Verification items for the finished model (mm, model axes). Face numbers are marked on the shaded views. A direction names the side the tool comes from. Coordinates: 2 decimals unless noted, no trailing zeros. Order: outer loops, then holes, each group sorted by start corner. A loop starts at its lowest first (then second) coordinate and runs counter-clockwise, first axis right, second up. Notation, with made-up numbers: (-9, -16) -> (15, -16) arc R12 cw to (15, -3) -> close; hole circle Ø5 at (80.5, 84.25). An arc over 180 degrees is marked (long way). Use CSV: the item, a comma, the result in double quotes. Start each with the question number.
1) Sectioned sample at D-D on z = -24. Record the boundary of the cut face in (x, y) (3 decimals).
2) Go/stop test with flat-tipped pins: pin 1 (4 mm diameter, centred on x = -39.5, y = 5.5, fed in from +Z); pin 2 (6.5 mm diameter, centred on x = -28, y = 9, fed in from -Z); pin 3 (19 mm diameter, centred on x = -19, z = -33.5, fed in from -Y); pin 4 (2 mm diameter, centred on x = -34, y = 9, fed in from -Z). Record where each tip stops, or that it passes through.
3) Release check for a two-part mould opening along X. For the marked faces 6, 7 and 8 record: released by +X, released by -X, zero draft, split by the parting line, or undercut.
4) Sectioned sample at A-A on z = 2.5. Record the boundary of the cut face in (x, y) (3 decimals), then the cut area to 3 significant figures.
5) Sectioned sample at C-C on y = 14. Record the boundary of the cut face in (x, z) (3 decimals), then the cut area to 3 significant figures.
6) Scan lines: line 1 along X through (y, z) = (8, -3) (3 decimals); line 2 along X through (y, z) = (8, 3.5) (3 decimals); line 3 along Y through (x, z) = (-34.5, -59.5) (3 decimals). Record each from-to range of solid material in increasing order.
7) Sectioned sample at B-B on x = -18. Record the boundary of the cut face in (y, z) (1 decimal).
8) Tool access check on the marked faces 1, 2, 3, 4 and 5. Record the directions out of +Z, -Z, +X, -X, +Y, -Y that give a thin tool (end or side, any length) a straight path to the whole face; none if there is none.
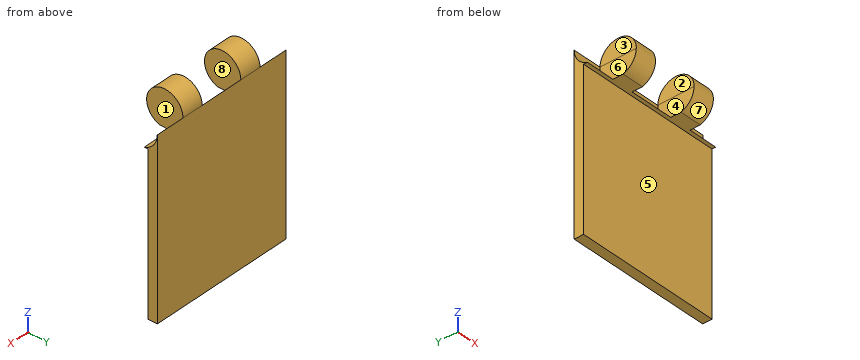
Autodesk Inventor part; units mm, degrees
ref_plane "XZ Plane" through (0, 0, 0) normal (0, 1, 0) x (-1, 0, 0)
ref_plane "XY Plane" through (0, 0, 0) normal (0, 0, 1) x (1, 0, 0)
sketch "Sketch1" plane through (0, 0, 0) normal (0, 1, 0) x (-1, 0, 0)
  line L0 (0, 0) -> (63.5, 0)
  line L1 (63.5, 0) -> (63.5, -76.2)
  line L2 (63.5, -76.2) -> (0, -76.2)
  line L3 (0, -76.2) -> (0, 0)
  dimension "d0" = 63.5
  dimension "d1" = 76.2
extrude "Extrusion1" add sketch "Sketch1" along normal blind 15.875
sketch "Sketch2" plane through (0, 0, 0) normal (1, 0, 0) x (0, 0, -1)
  line L0 (76.2, 0) -> (0, 0)
  line L1 (0, 0) -> (0, 15.875)
  circle A0 centre (0, 7.9375) radius 7.9375
  line L2 (76.2, 15.875) -> (0, 15.875)
extrude "Extrusion2" cut sketch "Sketch2" against normal blind 12.7 contours L1 A0 picked at (1.148, 10.3213)
ref_plane "Work Plane1" through (-31.75, 0, 0) normal (1, 0, 0) x (0, 1, 0)
mirror "Mirror1" about plane through (-31.75, 0, 0) normal (1, 0, 0) of "Extrusion2"
sketch "Sketch3" plane through (-12.7, 0, 0) normal (0, 0, 1) x (1, 0, 0)
  line L0 (12.7, 15.875) -> (-50.8, 15.875)
  line L1 (12.7, 0) -> (-50.8, 0)
  line L2 (-28.575, 15.875) -> (-9.525, 15.875)
  line L3 (-9.525, 15.875) -> (-9.525, 7.9375)
  line L4 (-28.575, 7.9375) -> (-28.575, 15.875)
  line L5 (0, 0) -> (0, 15.875)
  line L6 (-28.575, 7.9375) -> (-9.525, 7.9375)
  line L7 (-32.6367, 7.9375) -> (-5.0262, 7.9375)
  point P0 (-9.525, 15.875)
  dimension "d8" = 19.05
  dimension "d9" = 9.525
revolve "Revolution1" cut sketch "Sketch3" angle 360 about axis through (-45.3367, 7.9375, 0) along (1, 0, 0)
sketch "Sketch4" plane through (-12.7, 0, 0) normal (0, 0, 1) x (1, 0, 0)
  line L0 (12.7, 15.875) -> (-50.8, 15.875)
  line L1 (0, 0) -> (0, 15.875)
  line L2 (-9.4737, 15.875) -> (0, 15.875)
  line L3 (0, 15.875) -> (0, 7.9375)
  line L4 (0, 7.9375) -> (-9.4737, 7.9375)
  line L5 (-9.4737, 7.9375) -> (-9.4737, 15.875)
  line L6 (-28.575, 15.875) -> (-28.575, 0)
  line L7 (-38.032, 15.875) -> (-28.575, 15.875)
  line L8 (-28.575, 15.875) -> (-28.575, 7.9375)
  line L9 (-28.575, 7.9375) -> (-38.032, 7.9375)
  line L10 (-38.032, 7.9375) -> (-38.032, 15.875)
  line L11 (-38.032, 7.9375) -> (0, 7.9375)
  point P0 (12.7, 0)
revolve "Revolution2" add sketch "Sketch4" angle 360 about axis through (-50.732, 7.9375, 0) along (1, 0, 0) contours L1 L4 L5 L0 | L6 L9 L10 L0
sketch "Sketch5" plane through (0, 0, -76.2) normal (1, 0, 0) x (0, 0, -1)
  line L0 (0, 0) -> (0, 15.875)
  line L1 (0, 0) -> (-63.4859, 0)
  line L2 (-63.4859, 0) -> (-63.4859, -0.635)
  line L3 (-63.4859, -0.635) -> (0, -0.635)
  line L4 (0, -0.635) -> (0, 0)
  line L5 (-76.2, 15.875) -> (0, 15.875)
  point P0 (-76.2, 0)
  dimension "d12" = 16.51
extrude "Extrusion3" add sketch "Sketch5" against normal up to surface (63.5 mm away)
sketch "Sketch6" plane through (0, 7.9375, 0) normal (1, 0, 0) x (0, 0, -1)
  line L0 (12.7141, -8.5725) -> (76.2, -8.5725)
  line L1 (76.2, -8.5725) -> (7.62, -8.5725)
  line L2 (7.62, -8.5725) -> (7.62, 3.8481)
  line L3 (7.62, 3.8481) -> (76.2, 3.8481)
  line L4 (76.2, 3.8481) -> (76.2, -8.5725)
  line L5 (0, 7.9375) -> (76.2, 7.9375)
  point P0 (0, -7.9375)
  dimension "d15" = 4.0894
  dimension "d16" = 68.58
extrude "Extrusion4" cut sketch "Sketch6" against normal through all
sketch "Sketch7" plane through (0, 0, 0) normal (1, 0, 0) x (0, 0, -1)
  arc A0 (0, 0) -> (7.62, 5.715) centre (0, 7.9375) ccw
  line L0 (7.62, 5.715) -> (7.62, 0)
  line L1 (7.62, 0) -> (0, 0)
  arc A1 (0, 0) -> (7.62, 5.715) centre (0, 7.9375) ccw
extrude "Extrusion5" cut sketch "Sketch7" against normal through all
properties part number "knuckle plate hinge 2"
Answers follow:
1,outline,"(-63.5, 11.786) -> (0, 11.786) -> (0, 15.875) -> (-63.5, 15.875) -> close"
2,pin 1,"stops at z = 7.79"
2,pin 2,"stops at z = -76.2"
2,pin 3,"stops at y = 11.79"
2,pin 4,"passes through"
3,face 6,"released by -X"
3,face 7,"zero draft"
3,face 8,"undercut"
4,outline,"(-50.732, 0.404) -> (-41.275, 0.404) -> (-41.275, 15.471) -> (-50.732, 15.471) -> close; (-22.174, 0.404) -> (-12.7, 0.404) -> (-12.7, 15.471) -> (-22.174, 15.471) -> close"
4,area,"285 mm²"
5,outline,"(-63.5, -76.2) -> (0, -76.2) -> (0, -5.123) -> (-12.7, -5.123) -> (-12.7, 5.123) -> (-22.174, 5.123) -> (-22.174, 0) -> (-22.225, 0) -> (-22.225, -5.123) -> (-41.275, -5.123) -> (-41.275, 5.123) -> (-50.732, 5.123) -> (-50.732, 0) -> (-50.8, 0) -> (-50.8, -5.123) -> (-63.5, -5.123) -> close"
5,area,"4,710 mm²"
6,line 1,"x = -50.8 to -41.275, -22.225 to -12.7"
6,line 2,"x = -50.732 to -41.275, -22.174 to -12.7"
6,line 3,"y = 11.786 to 15.875"
7,outline,"(5.7, -7.6) -> (11.8, -7.6) -> (11.8, -76.2) -> (15.9, -76.2) -> (15.9, 0) arc R7.9 ccw (long way) to start"
8,face 1,"+Z, +X, -Y"
8,face 2,"+Z, +Y, -Y"
8,face 3,"+Z, -X, +Y, -Y"
8,face 4,"+Z, -Y"
8,face 5,"-Z, +X, -X, -Y"
